The listing builds one solid part. Answer for the finished solid, in the listing's coordinates (mm). A direction names the side the tool comes from. Round coordinates to 2 decimals unless told otherwise and drop trailing zeros. Order: outer loops, then holes, each group sorted by start corner. A loop starts at its lowest first (then second) coordinate and runs counter-clockwise, first axis right, second up. Notation, with made-up numbers: (-2.75, 3) - (20.25, 3) arc R25 cw to (20.25, 21) - close; hole circle Ø6 at (-37.75, -23.5). An arc over 180 degrees is marked (long way). One line per item, written item: value. Start each with the question number.
1. Section C-C, the plane x = 25 is taken. Give the vertices of the cut face in (y, z), then the cut area to 3 significant figures.
2. A tool of negligible diameter and unlimited length cuts with its end or side. For faces 5 (the cylindrical face through (12.911, -2.958, -6.535)), 6 (the flat face through (29.064, -13, -6)), from which of +Z, -Z, +X, -X, +Y, -Y can it reach the whole face along a straight path? Write none if from no direction.
3. Section D-D, the plane z = -3 is taken. Give the vertices of the cut face in (x, y), then the cut area to 3 significant figures.
4. Flat-ended cylindrical pins translate along their axes: P1, Ø3, axis at x = 23.5, z = -6.5, coming from the +Y side; P2, Ø4.5, axis at x = 21.06, z = -5.77, coming from the -Y side; P3, Ø4, axis at y = -16, z = -5.77, coming from the +X side. Find the tip coordinate at first contact, or state that the pin passes through.
5. Section B-B, the plane y = -16 is taken. Give the vertices of the cut face in (x, z), then the cut area to 3 significant figures.
6. Section A-A, the plane z = -5.25 is taken. Give the vertices of the cut face in (x, y).
7. For a pull along Z with two mould halves and no side action, classify faces 1 (the flat face through (23, -8, -13.769)), 2 (the cylindrical face through (19.066, -2.958, -5.681)), 3 (the cylindrical face through (32.11, -13.92, -6.63)), 4 (the flat face through (21.669, -13.605, -11.797)) as released by +Z, released by -Z, zero draft, split by the parting line, or undercut.
8. Straight lines are drawn through the part: line 1 (X direction, y = -4, z = -4.75); line 2 (Z direction, x = 32.45, y = -16); line 3 (Z direction, x = 19.5, y = -9.75). For each, find the intervals that lie inside material, in ascending order.
from build123d import *

# Parameters (mm, degrees)
F0_W     = 30
F0_H     = 16
F0_R     = 2
F1_DEPTH = 6
F2_W     = 6
F2_H     = 16
F3_DEPTH = 15
F5_DEPTH = 4
F7_DEPTH = 4
F8_R     = 2.25
F9_DEPTH = 25


with BuildPart() as f1:
    # F0 (on Front) → F1 (new body)
    with BuildSketch(Plane.XZ):
        with Locations((20.063871, -5.768647)):
            Rectangle(F0_W, F0_H)
        with Locations((11.063871, -5.768647)):
            Circle(F0_R, mode=Mode.SUBTRACT)
        with Locations((21.063871, -5.768647)):
            Circle(F0_R, mode=Mode.SUBTRACT)
    extrude(amount=F1_DEPTH)

    # F2 (on face) → F3 (join)
    with BuildSketch(Plane.XZ.offset(6)):
        with Locations((32.063871, -5.768647)):
            Rectangle(F2_W, F2_H)
    extrude(amount=F3_DEPTH)

    # F4 (on face) → F5 (join)
    with BuildSketch(Plane(origin=(0, 0, -13.768647), x_dir=(1, 0, 0), z_dir=(0, 0, -1))):
        Polygon((29.063871, 21), (14.063871, 6), (29.063871, 6), align=None)
    extrude(amount=-F5_DEPTH)

    # F6 (on face) → F7 (join)
    with BuildSketch(Plane.XY.offset(2.231353)):
        Polygon((29.063871, -21), (29.063871, -6), (14.063871, -6), align=None)
    extrude(amount=-F7_DEPTH)

    # F8 (on face) → F9 (cut)
    with BuildSketch(Plane.YZ.offset(35.063871)):
        with Locations((-16, -5.768647)):
            Circle(F8_R)
    extrude(amount=-F9_DEPTH, mode=Mode.SUBTRACT)


solid = f1.part
Answer list:
1. outline: (-16.94, -13.77) - (0, -13.77) - (0, 2.23) - (-16.94, 2.23) - (-16.94, -1.77) - (-6, -1.77) - (-6, -9.77) - (-16.94, -9.77) - close
1. area: 183 mm²
2. face 5: +Y, -Y
2. face 6: -X, -Y
3. outline: (5.06, -6) - (29.06, -6) - (29.06, -21) - (35.06, -21) - (35.06, 0) - (5.06, 0) - close
3. area: 270 mm²
4. P1: stops at y = 0
4. P2: stops at y = -6
4. P3: passes through
5. outline: (24.06, -13.77) - (35.06, -13.77) - (35.06, -8.02) - (29.06, -8.02) - (29.06, -9.77) - (24.06, -9.77) - close; (24.06, -1.77) - (29.06, -1.77) - (29.06, -3.52) - (35.06, -3.52) - (35.06, 2.23) - (24.06, 2.23) - close
5. area: 109 mm²
6. outline: (5.06, -6) - (9.13, -6) - (9.13, 0) - (5.06, 0) - close; (13, -6) - (19.13, -6) - (19.13, 0) - (13, 0) - close; (23, -6) - (29.06, -6) - (29.06, -13.81) - (35.06, -13.81) - (35.06, 0) - (23, 0) - close; (29.06, -21) - (35.06, -21) - (35.06, -18.19) - (29.06, -18.19) - close
7. face 1: released by -Z
7. face 2: undercut
7. face 3: undercut
7. face 4: zero draft
8. line 1: x = 5.06 to 9.34, 12.79 to 19.34, 22.79 to 35.06
8. line 2: z = -13.77 to -8.02, -3.52 to 2.23
8. line 3: z = -13.77 to -9.77, -1.77 to 2.23
